Here's the drawing with two shaded views (mm, measured from the low corner). I have some questions. Coordinates: 2 decimals unless noted, no trailing zeros. Write each loop counter-clockwise with the first axis right and the second up, starting at its lowest first coordinate (ties: lowest second). Pieces come first, ordered by that corner, then holes. Notation, with made-up numbers: (31.5, 33.25) -> (44.5, 33.25) arc R8 ccw to (44.5, 46.25) -> close; hole circle Ø9 at (-18, -31). An arc over 180 degrees is marked (long way). Put each result on its own line as item: value.
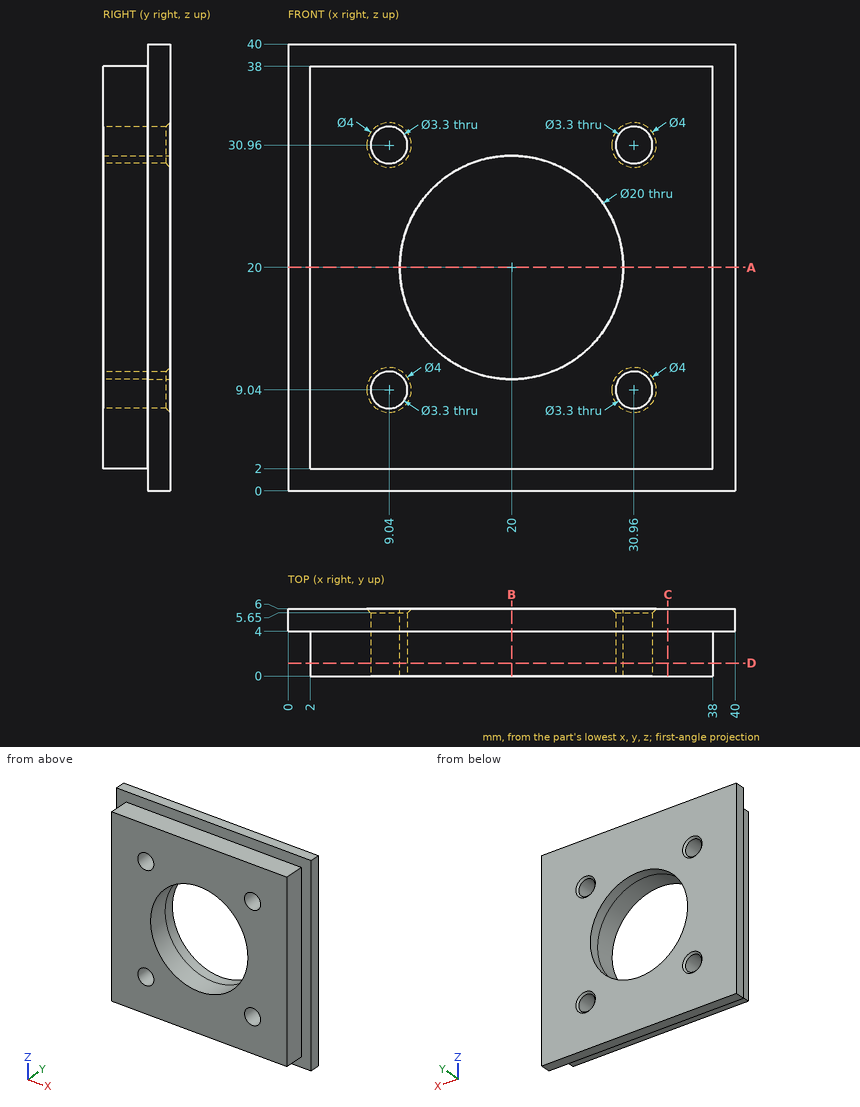
Item 1: Imagine slicing it at C-C on x = 34. Write out the boundary of the cut face in (y, z), then the cut area to 3 significant figures.
Output:
outline: (0, 2) -> (4, 2) -> (4, 0) -> (6, 0) -> (6, 40) -> (4, 40) -> (4, 38) -> (0, 38) -> close
area: 224 mm²
Item 2: For P1, Ø1, axis at y = 3, z = 28, coming from the +X side; P2, Ø3, axis at x = 32, y = 2, coming from the -Z side, each with a flat end and sliding along its axis, tell me the tip position at first contact or that it passes through.
Output:
P1: stops at x = 38
P2: stops at z = 2
Item 3: Imagine slicing it at A-A on z = 20. Write out the boundary of the cut face in (x, y).
Output:
outline: (0, 4) -> (2, 4) -> (2, 0) -> (10, 0) -> (10, 6) -> (0, 6) -> close; (30, 0) -> (38, 0) -> (38, 4) -> (40, 4) -> (40, 6) -> (30, 6) -> close
Item 4: Please list where these lines run through material, in increasing order: line 1 along X through (y, z) = (2.6, 20); line 2 along Z through (x, y) = (4, 3.9). Write a range as from..to.
Output:
line 1: x = 2..10, 30..38
line 2: z = 2..38
Item 5: Imagine slicing it at B-B on x = 20. Write out the boundary of the cut face in (y, z), then the cut area to 3 significant figures.
Output:
outline: (0, 2) -> (4, 2) -> (4, 0) -> (6, 0) -> (6, 10) -> (0, 10) -> close; (0, 30) -> (6, 30) -> (6, 40) -> (4, 40) -> (4, 38) -> (0, 38) -> close
area: 104 mm²
Item 6: Imagine slicing it at D-D on y = 1.15. Write out the boundary of the cut face in (x, z).
Output:
outline: (2, 2) -> (38, 2) -> (38, 38) -> (2, 38) -> close; hole circle Ø3.3 at (9.04, 9.04); hole circle Ø3.3 at (9.04, 30.96); hole circle Ø20 at (20, 20); hole circle Ø3.3 at (30.96, 9.04); hole circle Ø3.3 at (30.96, 30.96)
